Design review of the part built by this model. Coordinates are the model's own, in mm. Coordinates: 2 decimals unless noted, no trailing zeros. One line per question, with ' | ' between items. Start each with the question number.
Q1. Wall thickness on probe 1 along Z at (x, y) = (14, 11.5); probe 2 along Y at (x, z) = (8, 17) (3 decimals); probe 3 along X at (y, z) = (13, 4): over which ranges is each line inside the solid? List them lowest first.
Q2. Draft analysis for pull direction Y (two halves, no side actions). For faces 1 (the flat face through (-1, 0, 0)), 2 (the flat face through (-1, 0, 47)), 3 (the conical face through (59.89, -41.92, 44.96)), state which applies: pulls with the +Y half, pulls with the -Y half, needs draft (parallel to the pull), parting line crosses it, or undercut.
Q3. For P1, Ø1.1, axis at y = 5.5, z = 47.5, coming from the -X side; P2, Ø1.1, axis at y = 13.5, z = 47.5, coming from the +X side; P3, Ø1.5, axis at x = 14.5, y = 7, coming from the +Z side, all flat-tipped, find the tip position at first contact; note any pin that passes through.
from build123d import *

# Parameters (mm, degrees)
F0_W      = 111.22
F0_H      = 71.63
F2_W      = 121.14
F2_H      = 85.07
F4_R      = 5
F5_W      = 123.14
F5_H      = 87.07
F6_DEPTH  = 6
F7_W      = 101.22
F7_H      = 61.63
F8_DEPTH  = 1
F9_R      = 5
F10_SIZE2 = 5.99999
F10_SIZE  = 0.524922


# Not quite as in the source:
# - a fillet or chamfer is up to 0.001 mm smaller than in the source, because OpenCascade refuses the exact size


with BuildPart() as f3:
    # F0 (on Top) → F3 section 0
    with BuildSketch(Plane.XY):
        Rectangle(F0_W, F0_H)
    # F2 (on offset) → F3 section 1
    with BuildSketch(Plane.XY.offset(42)):
        Rectangle(F2_W, F2_H)
    loft()

    # F4
    f4_edges = [f3.edges().sort_by_distance(p)[0] for p in [
        (-55.61, 0, 0),
        (-58.09, 39.175, 21),
        (0, 35.815, 0),
        (55.61, 0, 0),
        (58.09, 39.175, 21),
        (-58.09, -39.175, 21),
        (0, -35.815, 0),
        (58.09, -39.175, 21),
    ]]
    fillet(f4_edges, radius=F4_R)

    # F5 (on face) → F6 (join)
    with BuildSketch(Plane.XY.offset(42)):
        Rectangle(F5_W, F5_H)
        with BuildLine():
            Line((60.57, 37.5652286365), (60.57, -37.5652286365))
            add(Edge.make_bspline(
                [(60.57, -37.5652286365), (60.57, -37.8677629795), (60.5484249291, -38.1785474247), (60.5029654317, -38.4950915318), (60.4316524162, -38.8141360023), (60.3333363666, -39.1316751054), (60.0821499269, -39.7565973164), (59.9290553292, -40.0639382754), (59.7486936762, -40.3612591505), (59.5421641644, -40.6440796366), (59.3119172372, -40.9083408285), (58.8238966802, -41.3807158702), (58.5682195509, -41.5910650721), (58.2970619174, -41.7793580892), (58.013945443, -41.9437291503), (57.7226574277, -42.0834034649), (57.1273207787, -42.3149957608), (56.8231561933, -42.4063160322), (56.5180078096, -42.4725842951), (56.2153860403, -42.5148862736), (55.9181609136, -42.535), (55.628544141, -42.535)],
                knots=[0, 0, 0, 0, 0, 0, 0, 0.2552622354, 0.2552622354, 0.2552622354, 0.2552622354, 0.2552622354, 0.5115672797, 0.5115672797, 0.5115672797, 0.5115672797, 0.5115672797, 0.7543107062, 0.7543107062, 0.7543107062, 0.7543107062, 0.7543107062, 1, 1, 1, 1, 1, 1, 1], degree=6))
            Line((55.628544141, -42.535), (-55.628544141, -42.535))
            add(Edge.make_bspline(
                [(-60.57, -37.5652286365), (-60.57, -37.8677629794), (-60.5484249292, -38.1785474246), (-60.5029654317, -38.4950915316), (-60.4316524163, -38.814136002), (-60.3333363667, -39.1316751051), (-60.0821499271, -39.756597316), (-59.9290553294, -40.0639382751), (-59.7486936764, -40.3612591501), (-59.5421641646, -40.6440796363), (-59.3119172375, -40.9083408282), (-58.8238966804, -41.38071587), (-58.5682195512, -41.591065072), (-58.2970619176, -41.7793580891), (-58.0139454431, -41.9437291502), (-57.7226574278, -42.0834034648), (-57.1273207787, -42.3149957608), (-56.8231561933, -42.4063160322), (-56.5180078096, -42.4725842951), (-56.2153860403, -42.5148862736), (-55.9181609136, -42.535), (-55.628544141, -42.535)],
                knots=[0, 0, 0, 0, 0, 0, 0, 0.2552622353, 0.2552622353, 0.2552622353, 0.2552622353, 0.2552622353, 0.5115672797, 0.5115672797, 0.5115672797, 0.5115672797, 0.5115672797, 0.7543107062, 0.7543107062, 0.7543107062, 0.7543107062, 0.7543107062, 1, 1, 1, 1, 1, 1, 1], degree=6))
            Line((-60.57, -37.5652286365), (-60.57, 37.5652286365))
            add(Edge.make_bspline(
                [(-55.628544141, 42.535), (-55.9165579294, 42.535), (-56.2120960387, 42.5151083241), (-56.5129833201, 42.4732846379), (-56.8164007689, 42.4077788273), (-57.1189028719, 42.3175153178), (-57.7138767296, 42.0875473103), (-58.0063798227, 41.9479897602), (-58.2907253957, 41.7835490477), (-58.5630840084, 41.5949938834), (-58.8198912965, 41.3842007295), (-59.3081604347, 40.9123831651), (-59.5378156039, 40.6494264179), (-59.7439719788, 40.3680131083), (-59.924197311, 40.0721470067), (-60.0773872558, 39.7662523131), (-60.3304237584, 39.1410513034), (-60.4299622755, 38.821673494), (-60.5021575431, 38.500700594), (-60.5481693204, 38.1822186305), (-60.57, 37.8695496868), (-60.57, 37.5652286365)],
                knots=[0, 0, 0, 0, 0, 0, 0, 0.2443294294, 0.2443294294, 0.2443294294, 0.2443294294, 0.2443294294, 0.4879249993, 0.4879249993, 0.4879249993, 0.4879249993, 0.4879249993, 0.7432302237, 0.7432302237, 0.7432302237, 0.7432302237, 0.7432302237, 1, 1, 1, 1, 1, 1, 1], degree=6))
            Line((-55.628544141, 42.535), (55.628544141, 42.535))
            add(Edge.make_bspline(
                [(60.57, 37.5652286365), (60.57, 37.8677629794), (60.5484249292, 38.1785474246), (60.5029654317, 38.4950915316), (60.4316524163, 38.814136002), (60.3333363667, 39.1316751051), (60.0821499271, 39.756597316), (59.9290553294, 40.0639382751), (59.7486936764, 40.3612591501), (59.5421641646, 40.6440796363), (59.3119172375, 40.9083408282), (58.8238966804, 41.38071587), (58.5682195512, 41.591065072), (58.2970619176, 41.7793580891), (58.0139454431, 41.9437291502), (57.7226574278, 42.0834034648), (57.1273207787, 42.3149957608), (56.8231561933, 42.4063160322), (56.5180078096, 42.4725842951), (56.2153860403, 42.5148862736), (55.9181609136, 42.535), (55.628544141, 42.535)],
                knots=[0, 0, 0, 0, 0, 0, 0, 0.2552622353, 0.2552622353, 0.2552622353, 0.2552622353, 0.2552622353, 0.5115672797, 0.5115672797, 0.5115672797, 0.5115672797, 0.5115672797, 0.7543107062, 0.7543107062, 0.7543107062, 0.7543107062, 0.7543107062, 1, 1, 1, 1, 1, 1, 1], degree=6))
        make_face(mode=Mode.SUBTRACT)
        with BuildLine():
            add(Edge.make_bspline(
                [(60.57, -37.5652286365), (60.57, -37.8677629795), (60.5484249291, -38.1785474247), (60.5029654317, -38.4950915318), (60.4316524162, -38.8141360023), (60.3333363666, -39.1316751054), (60.0821499269, -39.7565973164), (59.9290553292, -40.0639382754), (59.7486936762, -40.3612591505), (59.5421641644, -40.6440796366), (59.3119172372, -40.9083408285), (58.8238966802, -41.3807158702), (58.5682195509, -41.5910650721), (58.2970619174, -41.7793580892), (58.013945443, -41.9437291503), (57.7226574277, -42.0834034649), (57.1273207787, -42.3149957608), (56.8231561933, -42.4063160322), (56.5180078096, -42.4725842951), (56.2153860403, -42.5148862736), (55.9181609136, -42.535), (55.628544141, -42.535)],
                knots=[0, 0, 0, 0, 0, 0, 0, 0.2552622354, 0.2552622354, 0.2552622354, 0.2552622354, 0.2552622354, 0.5115672797, 0.5115672797, 0.5115672797, 0.5115672797, 0.5115672797, 0.7543107062, 0.7543107062, 0.7543107062, 0.7543107062, 0.7543107062, 1, 1, 1, 1, 1, 1, 1], degree=6))
            Line((60.57, -37.5652286365), (60.57, 37.5652286365))
            add(Edge.make_bspline(
                [(60.57, 37.5652286365), (60.57, 37.8677629794), (60.5484249292, 38.1785474246), (60.5029654317, 38.4950915316), (60.4316524163, 38.814136002), (60.3333363667, 39.1316751051), (60.0821499271, 39.756597316), (59.9290553294, 40.0639382751), (59.7486936764, 40.3612591501), (59.5421641646, 40.6440796363), (59.3119172375, 40.9083408282), (58.8238966804, 41.38071587), (58.5682195512, 41.591065072), (58.2970619176, 41.7793580891), (58.0139454431, 41.9437291502), (57.7226574278, 42.0834034648), (57.1273207787, 42.3149957608), (56.8231561933, 42.4063160322), (56.5180078096, 42.4725842951), (56.2153860403, 42.5148862736), (55.9181609136, 42.535), (55.628544141, 42.535)],
                knots=[0, 0, 0, 0, 0, 0, 0, 0.2552622353, 0.2552622353, 0.2552622353, 0.2552622353, 0.2552622353, 0.5115672797, 0.5115672797, 0.5115672797, 0.5115672797, 0.5115672797, 0.7543107062, 0.7543107062, 0.7543107062, 0.7543107062, 0.7543107062, 1, 1, 1, 1, 1, 1, 1], degree=6))
            Line((55.628544141, 42.535), (-55.628544141, 42.535))
            add(Edge.make_bspline(
                [(-55.628544141, 42.535), (-55.9165579294, 42.535), (-56.2120960387, 42.5151083241), (-56.5129833201, 42.4732846379), (-56.8164007689, 42.4077788273), (-57.1189028719, 42.3175153178), (-57.7138767296, 42.0875473103), (-58.0063798227, 41.9479897602), (-58.2907253957, 41.7835490477), (-58.5630840084, 41.5949938834), (-58.8198912965, 41.3842007295), (-59.3081604347, 40.9123831651), (-59.5378156039, 40.6494264179), (-59.7439719788, 40.3680131083), (-59.924197311, 40.0721470067), (-60.0773872558, 39.7662523131), (-60.3304237584, 39.1410513034), (-60.4299622755, 38.821673494), (-60.5021575431, 38.500700594), (-60.5481693204, 38.1822186305), (-60.57, 37.8695496868), (-60.57, 37.5652286365)],
                knots=[0, 0, 0, 0, 0, 0, 0, 0.2443294294, 0.2443294294, 0.2443294294, 0.2443294294, 0.2443294294, 0.4879249993, 0.4879249993, 0.4879249993, 0.4879249993, 0.4879249993, 0.7432302237, 0.7432302237, 0.7432302237, 0.7432302237, 0.7432302237, 1, 1, 1, 1, 1, 1, 1], degree=6))
            Line((-60.57, 37.5652286365), (-60.57, -37.5652286365))
            add(Edge.make_bspline(
                [(-60.57, -37.5652286365), (-60.57, -37.8677629794), (-60.5484249292, -38.1785474246), (-60.5029654317, -38.4950915316), (-60.4316524163, -38.814136002), (-60.3333363667, -39.1316751051), (-60.0821499271, -39.756597316), (-59.9290553294, -40.0639382751), (-59.7486936764, -40.3612591501), (-59.5421641646, -40.6440796363), (-59.3119172375, -40.9083408282), (-58.8238966804, -41.38071587), (-58.5682195512, -41.591065072), (-58.2970619176, -41.7793580891), (-58.0139454431, -41.9437291502), (-57.7226574278, -42.0834034648), (-57.1273207787, -42.3149957608), (-56.8231561933, -42.4063160322), (-56.5180078096, -42.4725842951), (-56.2153860403, -42.5148862736), (-55.9181609136, -42.535), (-55.628544141, -42.535)],
                knots=[0, 0, 0, 0, 0, 0, 0, 0.2552622353, 0.2552622353, 0.2552622353, 0.2552622353, 0.2552622353, 0.5115672797, 0.5115672797, 0.5115672797, 0.5115672797, 0.5115672797, 0.7543107062, 0.7543107062, 0.7543107062, 0.7543107062, 0.7543107062, 1, 1, 1, 1, 1, 1, 1], degree=6))
            Line((-55.628544141, -42.535), (55.628544141, -42.535))
        make_face()
    extrude(amount=F6_DEPTH)

    # F7 (on face) → F8 (cut)
    with BuildSketch(Plane.XY.offset(48)):
        Rectangle(F7_W, F7_H)
    extrude(amount=-F8_DEPTH, mode=Mode.SUBTRACT)

    # F9
    f9_edges = [f3.edges().sort_by_distance(p)[0] for p in [
        (-61.57, 43.535, 45),
        (-61.57, -43.535, 45),
        (61.57, -43.535, 45),
        (61.57, 43.535, 45),
    ]]
    fillet(f9_edges, radius=F9_R)

    # F10 (size 0.5249319812 and 6 in the source; OpenCascade refuses exactly that, so slightly less here)
    f10_edges = [f3.edges().sort_by_distance(p)[0] for p in [
        (61.57, 0, 48),
        (60.105534, 42.070534, 48),
        (0, 43.535, 48),
        (-60.105534, 42.070534, 48),
        (-61.57, 0, 48),
        (-60.105534, -42.070534, 48),
        (0, -43.535, 48),
        (60.105534, -42.070534, 48),
    ]]
    f10_side = f3.faces().sort_by_distance((60.061867, 0, 48))[0]
    chamfer(f10_edges, length=F10_SIZE, length2=F10_SIZE2, reference=f10_side)


solid = f3.part
Output values:
1) probe 1: z = 0 to 47 | probe 2: y = -38.535 to 38.535 | probe 3: x = -56.06 to 56.06
2) face 1: needs draft | face 2: undercut | face 3: pulls with the -Y half
3) P1: stops at x = -61.14 | P2: stops at x = 61.14 | P3: stops at z = 47
